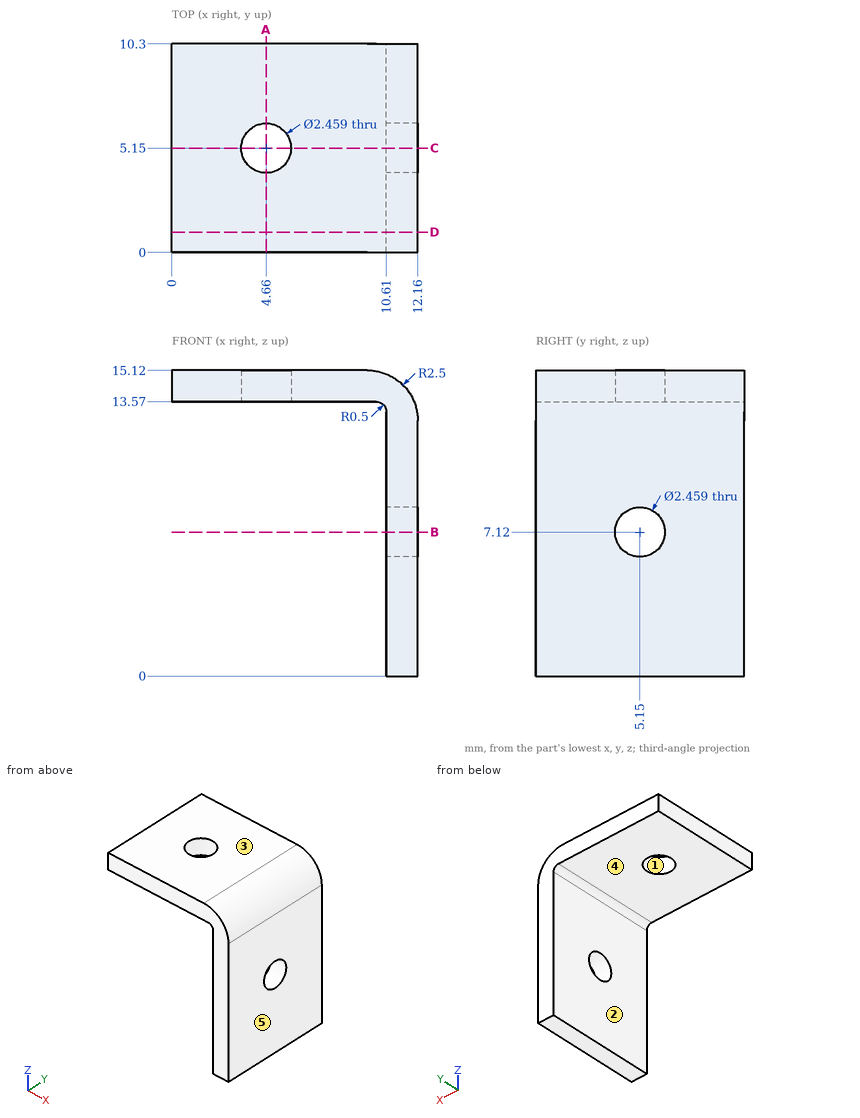
Design review of the part shown in the three views and the two pictorial views. Dimensions are in mm from the part's minimum x, y and z. A direction names the side the tool comes from. Coordinates: 2 decimals unless noted, no trailing zeros. Write each loop counter-clockwise with the first axis right and the second up, starting at its lowest first coordinate (ties: lowest second). Pieces come first, ordered by that corner, then holes.
(1) Tool access review of the marked faces 4 and 5: name each direction out of +Z, -Z, +X, -X, +Y, -Y from which nothing blocks a thin tool from reaching the whole face with its end or side.
(2) Wall thickness on probe 1 along Y at (x, z) = (4.66, 14); probe 2 along X at (y, z) = (7, 9.75); probe 3 along Z at (x, y) = (2.5, 8.5): over which ranges is each line inside the solid? List them lowest first.
(3) Add section A-A on x = 4.66. Give the boundary of the cut face in (y, z).
(4) Add section D-D on y = 1. Give the boundary of the cut face in (x, z), then the cut area to 3 significant figures.
(5) Add section B-B on z = 7.12. Give the boundary of the cut face in (x, y).
(6) Add section C-C on y = 5.15. Give the boundary of the cut face in (x, z).
(7) The part is to be moulded in two halves that separate along X. For the marked faces 1, 2 and 3, say which applies: +X half, -X half, draft (parallel to the pull), parting line (faces both ways), or undercut.
(8) For pin 1 Ø4 at (y, z) = (5.15, 7.12) entering from +X; pin 2 Ø5 at (x, y) = (3.5, 7.5) entering from -Z; pin 3 Ø5 at (y, z) = (7.5, 7) entering from -X, all flat-tipped, find the tip position at first contact; note any pin that passes through.
Answer sheet:
1. face 4: -Z, -X, +Y, -Y
1. face 5: +Z, -Z, +X, +Y, -Y
2. probe 1: y = 0 to 3.92, 6.38 to 10.3
2. probe 2: x = 10.61 to 12.16
2. probe 3: z = 13.57 to 15.12
3. outline: (0, 13.57) - (3.92, 13.57) - (3.92, 15.12) - (0, 15.12) - close; (6.38, 13.57) - (10.3, 13.57) - (10.3, 15.12) - (6.38, 15.12) - close
4. outline: (0, 13.57) - (10.11, 13.57) arc R0.5 cw to (10.61, 13.07) - (10.61, 0) - (12.16, 0) - (12.16, 12.62) arc R2.5 ccw to (9.66, 15.12) - (0, 15.12) - close
4. area: 38.6 mm2
5. outline: (10.61, 0) - (12.16, 0) - (12.16, 3.92) - (10.61, 3.92) - close; (10.61, 6.38) - (12.16, 6.38) - (12.16, 10.3) - (10.61, 10.3) - close
6. outline: (0, 13.57) - (3.43, 13.57) - (3.43, 15.12) - (0, 15.12) - close; (5.89, 13.57) - (10.11, 13.57) arc R0.5 cw to (10.61, 13.07) - (10.61, 8.35) - (12.16, 8.35) - (12.16, 12.62) arc R2.5 ccw to (9.66, 15.12) - (5.89, 15.12) - close; (10.61, 0) - (12.16, 0) - (12.16, 5.89) - (10.61, 5.89) - close
7. face 1: undercut
7. face 2: -X half
7. face 3: draft
8. pin 1: stops at x = 12.16
8. pin 2: stops at z = 13.57
8. pin 3: stops at x = 10.61
